```python
from build123d import *

# Parameters (mm, degrees)
BOSS_EXTRUDE1_DEPTH = 20
CUT_EXTRUDE2_START  = -10
CUT_EXTRUDE2_DEPTH  = 10


with BuildPart() as part:
    # Sketch1 → Boss-Extrude1 (new body)
    with BuildSketch(Plane.XY):
        with BuildLine():
            Line((106.370051436, 5.820149254), (-10.169418344, 5.820149254))
            ThreePointArc((-10.169418344, 5.820149254), (-14.260240152, 29.162077744), (-15.629948564, 52.820149254))
            Line((-15.629948564, 52.820149254), (-30.629948564, 52.820149254))
            ThreePointArc((-30.629948564, 52.820149254), (189.370051436, -167.179850746), (409.370051436, 52.820149254))
            Line((409.370051436, 52.820149254), (394.370051436, 52.820149254))
            ThreePointArc((394.370051436, 52.820149254), (393.000343025, 29.162077744), (388.909521216, 5.820149254))
            Line((388.909521216, 5.820149254), (272.370051436, 5.820149254))
            Line((272.370051436, 5.820149254), (272.370051436, -19.179850746))
            Line((272.370051436, -19.179850746), (252.670051436, -19.179850746))
            Line((252.670051436, -19.179850746), (252.670051436, -59.179850746))
            Line((252.670051436, -59.179850746), (249.070051436, -59.179850746))
            Line((249.070051436, -59.179850746), (249.070051436, -19.179850746))
            Line((249.070051436, -19.179850746), (229.370051436, -19.179850746))
            Line((229.370051436, -19.179850746), (229.370051436, -82.179850746))
            Line((229.370051436, -82.179850746), (149.370051436, -82.179850746))
            Line((149.370051436, -82.179850746), (149.370051436, -19.179850746))
            Line((149.370051436, -19.179850746), (129.670051436, -19.179850746))
            Line((129.670051436, -19.179850746), (129.670051436, -59.179850746))
            Line((129.670051436, -59.179850746), (126.070051436, -59.179850746))
            Line((126.070051436, -59.179850746), (126.070051436, -19.179850746))
            Line((126.070051436, -19.179850746), (106.370051436, -19.179850746))
            Line((106.370051436, -19.179850746), (106.370051436, 5.820149254))
        make_face()
    extrude(amount=BOSS_EXTRUDE1_DEPTH)

    # Sketch2 → Cut-Extrude2 (cut)
    with BuildSketch(Plane.XY.offset(20).offset(CUT_EXTRUDE2_START)):
        with BuildLine():
            Line((-10.169418344, 5.820149254), (106.370051436, 5.820149254))
            Line((106.370051436, 5.820149254), (106.370051436, -19.179850746))
            Line((106.370051436, -19.179850746), (126.070051436, -19.179850746))
            Line((126.070051436, -19.179850746), (126.070051436, -59.179850746))
            Line((126.070051436, -59.179850746), (129.670051436, -59.179850746))
            Line((129.670051436, -59.179850746), (129.670051436, -19.179850746))
            Line((129.670051436, -19.179850746), (149.370051436, -19.179850746))
            Line((149.370051436, -19.179850746), (149.370051436, -82.179850746))
            Line((149.370051436, -82.179850746), (229.370051436, -82.179850746))
            Line((229.370051436, -82.179850746), (229.370051436, -19.179850746))
            Line((229.370051436, -19.179850746), (249.070051436, -19.179850746))
            Line((249.070051436, -19.179850746), (249.070051436, -59.179850746))
            Line((249.070051436, -59.179850746), (252.670051436, -59.179850746))
            Line((252.670051436, -59.179850746), (252.670051436, -19.179850746))
            Line((252.670051436, -19.179850746), (272.370051436, -19.179850746))
            Line((272.370051436, -19.179850746), (272.370051436, 5.820149254))
            Line((272.370051436, 5.820149254), (388.909521216, 5.820149254))
            ThreePointArc((388.909521216, 5.820149254), (189.370051436, -152.179850746), (-10.169418344, 5.820149254))
        make_face()
    extrude(amount=CUT_EXTRUDE2_DEPTH, mode=Mode.SUBTRACT)


solid = part.part
```
Check sheet for the modelled part. Datum: model origin and axes. Units: mm. A direction names the side the tool comes from. Round coordinates to 2 decimals unless told otherwise and drop trailing zeros. Loops run counter-clockwise (first coordinate to the right, second up) from the corner with the lowest first, then second, coordinate; pieces in that order, holes last. Notation, with made-up numbers: M 87.25,81.5 L 126.25,81.5 A16 cw 126.25,91.5 Z; hole C 34,47 d11. An arc over 180 degrees is marked long. Answer as a JSON object with one key per item and string values.
1. Access from +Z, -Z, +X, -X, +Y, -Y to the whole of each face (thin tool, end or side, straight path). Record for faces 4 (the flat face through (192, -90, 10)), 5 (the flat face through (-23, 52.82, 10)), 6 (the flat face through (229.37, -50, 5)).
Reply:
{"face 4": "+Z, +Y", "face 5": "+Z, -Z, +X, -X, +Y", "face 6": "+Z, -Z, +Y"}
2. Gauge pin test, flat ends, axial feed: P1, Ø11, axis at y = -5.5, z = 7.5, coming from the +X side; P2, Ø5, axis at x = 324.5, z = 4, coming from the +Y side; P3, Ø6, axis at y = -84, z = 11, coming from the -X side. Record the tip position at first contact, or that the pin passes through.
Reply:
{"P1": "stops at x = 402.94", "P2": "stops at y = 5.82", "P3": "stops at x = 14.75"}
3. Section check B-B (z = 4.75). Record the boundary of the cut face in (x, y), plus the area to 3 significant figures.
Reply:
{"outline": "M -30.63,52.82 A220 ccw 409.37,52.82 L 394.37,52.82 A205 cw 388.91,5.82 L 272.37,5.82 L 272.37,-19.18 L 252.67,-19.18 L 252.67,-59.18 L 249.07,-59.18 L 249.07,-19.18 L 229.37,-19.18 L 229.37,-82.18 L 149.37,-82.18 L 149.37,-19.18 L 129.67,-19.18 L 129.67,-59.18 L 126.07,-59.18 L 126.07,-19.18 L 106.37,-19.18 L 106.37,5.82 L -10.17,5.82 A205 cw -15.63,52.82 Z", "area": "47,400 mm²"}
4. Section check C-C (y = -114.5). Record the boundary of the cut face in (x, z).
Reply:
{"outline": "M 46.53,0 L 332.21,0 L 332.21,20 L 307.81,20 L 307.81,10 L 70.93,10 L 70.93,20 L 46.53,20 Z"}
5. Mould release check, pull along X, two halves, no side actions. Record for faces 1 (the flat face through (188, -154, 20)), 2 (the flat face through (272.37, -7, 5)), 3 (the cylindrical face through (184.532, -167.127, 9.86)): pulls with the +X half, pulls with the -X half, needs draft (parallel to the pull), parting line crosses it, or undercut.
Reply:
{"face 1": "needs draft", "face 2": "undercut", "face 3": "parting line crosses it"}
6. Scan lines: line 1 (X direction, y = -45, z = 7.75); line 2 (X direction, y = -59, z = 2.25); line 3 (Z direction, x = 137.5, y = -126). Record each from-to range of solid material in increasing order.
Reply:
{"line 1": "x = -7.69 to 126.07, 129.67 to 149.37, 229.37 to 249.07, 252.67 to 386.43", "line 2": "x = -0.09 to 126.07, 129.67 to 149.37, 229.37 to 249.07, 252.67 to 378.83", "line 3": "z = 0 to 10"}
7. Section check A-A (y = -47). Record the boundary of the cut face in (x, z).
Reply:
{"outline": "M -6.68,0 L 126.07,0 L 126.07,10 L 10.31,10 L 10.31,20 L -6.68,20 Z; M 129.67,0 L 149.37,0 L 149.37,10 L 129.67,10 Z; M 229.37,0 L 249.07,0 L 249.07,10 L 229.37,10 Z; M 252.67,0 L 385.42,0 L 385.42,20 L 368.43,20 L 368.43,10 L 252.67,10 Z"}
8. Section check D-D (x = 4). Record the boundary of the cut face in (y, z), plus the area to 3 significant figures.
Reply:
{"outline": "M -65.66,0 L 5.82,0 L 5.82,10 L -34.72,10 L -34.72,20 L -65.66,20 Z", "area": "1,020 mm²"}
